```python
from build123d import *

# Parameters (mm, degrees)
BOSS_EXTRUDE1_DEPTH                                  = 4.7625
CUT_EXTRUDE2_DEPTH                                   = 349.730645664
CSK_FOR_M5_CROSS_RECESS_FLAT_HEAD_SCREW1_D           = 3.9624
CSK_FOR_M5_CROSS_RECESS_FLAT_HEAD_SCREW1_CSINK_D     = 6.35
CSK_FOR_M5_CROSS_RECESS_FLAT_HEAD_SCREW1_CSINK_ANGLE = 60
CIRPATTERN1_COUNT                                    = 19
CIRPATTERN1_ANGLE                                    = 45
CBORE_FOR_M5_CROSS_RECESS_PAN_HEAD_SCREW_D           = 4.3434
CBORE_FOR_M5_CROSS_RECESS_PAN_HEAD_SCREW_CBORE_D     = 7.9502
CBORE_FOR_M5_CROSS_RECESS_PAN_HEAD_SCREW_CBORE_DEPTH = 4.1656
CUT_EXTRUDE5_DEPTH                                   = 3.175
F_1_4_20_TAPPED_HOLE1_D                              = 5.1054
F_1_4_20_TAPPED_HOLE1_DEPTH                          = 19.05
F_1_4_20_TAPPED_HOLE1_CSINK_D                        = 7.62
F_1_4_20_TAPPED_HOLE1_CSINK_ANGLE                    = 90
F_1_4_20_TAPPED_HOLE1_TIP                            = 1.533816902


with BuildPart() as part:
    # Sketch1 → Boss-Extrude1 (new, symmetric)
    with BuildSketch(Plane(origin=(0, 0, 0), x_dir=(1, 0, 0), z_dir=(0, 1, 0))):
        with BuildLine():
            Line((38.1, 86.658308315), (238.76, 86.658308315))
            ThreePointArc((238.76, 86.658308315), (135.186201707, 215.036487295), (-25.4, 252.726809025))
            Line((-25.4, 252.726809025), (-25.4, 196.85))
            Line((-25.4, 196.85), (38.1, 133.35))
            Line((38.1, 133.35), (38.1, 86.658308315))
        make_face()
    extrude(amount=BOSS_EXTRUDE1_DEPTH, both=True)

    # Sketch2 → Cut-Extrude2 (cut, through all)
    with BuildSketch(Plane(origin=(0, 4.7625, 0), x_dir=(1, 0, 0), z_dir=(0, 1, 0))):
        with BuildLine():
            ThreePointArc((180.827242585, 147.531326552), (107.760674963, 207.006330595), (17.132342345, 232.74549796))
            ThreePointArc((17.132342345, 232.74549796), (11.965081824, 228.286801882), (16.423777903, 223.119541362))
            ThreePointArc((16.423777903, 223.119541362), (103.303877349, 198.444902033), (173.348536427, 141.429682659))
            ThreePointArc((173.348536427, 141.429682659), (180.138711452, 140.741151526), (180.827242585, 147.531326552))
        make_face()
    extrude(amount=-CUT_EXTRUDE2_DEPTH, mode=Mode.SUBTRACT)

    # CSK for M5 Cross Recess Flat Head Screw1 (through all)
    with Locations(Plane(origin=(0, -4.7625, 0), x_dir=(-1, 0, 0), z_dir=(0, -1, 0))):
        with Locations((-42.342371642, 240.135522494)):
            csk_for_m5_cross_recess_flat_head_screw1 = CounterSinkHole(CSK_FOR_M5_CROSS_RECESS_FLAT_HEAD_SCREW1_D / 2, CSK_FOR_M5_CROSS_RECESS_FLAT_HEAD_SCREW1_CSINK_D / 2, counter_sink_angle=CSK_FOR_M5_CROSS_RECESS_FLAT_HEAD_SCREW1_CSINK_ANGLE)

    # CirPattern1: CSK for M5 Cross Recess Flat Head Screw1 ×19 about axis
    cirpattern1_axis = Axis((0, 0, 0), (0, -1, 0))
    for i in range(1, CIRPATTERN1_COUNT):
        add(csk_for_m5_cross_recess_flat_head_screw1.rotate(cirpattern1_axis, i * CIRPATTERN1_ANGLE / (CIRPATTERN1_COUNT - 1)), mode=Mode.SUBTRACT)

    # CBORE for M5 Cross Recess Pan Head Screw2 (through all)
    with Locations(Plane(origin=(0, -4.7625, 0), x_dir=(-1, 0, 0), z_dir=(0, -1, 0))):
        with Locations((-45.72, 192.1002), (-45.72, 109.5502)):
            CounterBoreHole(CBORE_FOR_M5_CROSS_RECESS_PAN_HEAD_SCREW_D / 2, CBORE_FOR_M5_CROSS_RECESS_PAN_HEAD_SCREW_CBORE_D / 2, CBORE_FOR_M5_CROSS_RECESS_PAN_HEAD_SCREW_CBORE_DEPTH)

    # Sketch10 → Cut-Extrude5 (cut)
    with BuildSketch(Plane(origin=(0, 4.7625, 0), x_dir=(1, 0, 0), z_dir=(0, 1, 0))):
        with BuildLine():
            Line((203.2, 94.532308315), (203.2, 86.658308315))
            Line((203.2, 86.658308315), (212.852, 86.658308315))
            Line((212.852, 86.658308315), (212.852, 94.532308315))
            ThreePointArc((212.852, 94.532308315), (208.026, 99.358308315), (203.2, 94.532308315))
        make_face()
    extrude(amount=-CUT_EXTRUDE5_DEPTH, mode=Mode.SUBTRACT)

    # 1/4-20 Tapped Hole1
    with Locations(Plane.XY.offset(-86.658308315)):
        with Locations((64.77, 0), (144.145, 0), (223.52, 0)):
            CounterSinkHole(F_1_4_20_TAPPED_HOLE1_D / 2, F_1_4_20_TAPPED_HOLE1_CSINK_D / 2, depth=F_1_4_20_TAPPED_HOLE1_DEPTH, counter_sink_angle=F_1_4_20_TAPPED_HOLE1_CSINK_ANGLE)
            with Locations((0, 0, -(F_1_4_20_TAPPED_HOLE1_DEPTH + F_1_4_20_TAPPED_HOLE1_TIP / 2))):  # 118° drill point
                Cone(0, F_1_4_20_TAPPED_HOLE1_D / 2, F_1_4_20_TAPPED_HOLE1_TIP, mode=Mode.SUBTRACT)


solid = part.part
```
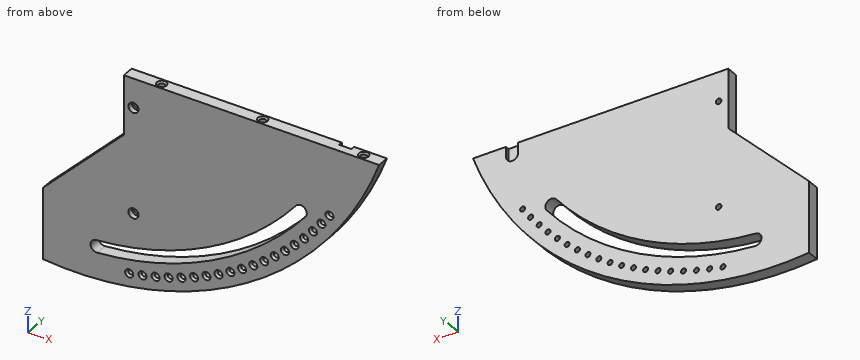
Here's how the part is built. I have some questions about the finished solid (model axes, mm). Coordinates: 2 decimals unless noted, no trailing zeros. Write each loop counter-clockwise with the first axis right and the second up, starting at its lowest first coordinate (ties: lowest second). Pieces come first, ordered by that corner, then holes. Notation, with made-up numbers: M 55,57 L 111,57 A28 ccw 111,82 Z; hole C 44.5,78.25 d5. An arc over 180 degrees is marked long. Answer as CSV lines item,"result". Start each with the question number.
Q1. Will these pins go through, and if not, where does the flat tip stop? pin 1 Ø4.5 at (x, z) = (164.74, -179.78) entering from -Y; pin 2 Ø3 at (x, z) = (206.5, -93) entering from +Y; pin 3 Ø5 at (x, z) = (73.32, -232.55) entering from -Y.
Q2. I need wall thicknesses on probe 1 along Z at (x, y) = (172.5, -0.75); probe 2 along Z at (x, y) = (122, 3); probe 3 along X at (y, z) = (-1.75, -180). Which ranges of each line are inside material? Lowest first, please. Write a range as [from, to].
Q3. Suppose I cut it at A-A, the plane z = -121. List the corners of the cut face in (x, y) for me, then the cut area to 3 significant figures.
Entries:
1,pin 1,"stops at y = -3.17"
1,pin 2,"stops at y = 1.59"
1,pin 3,"stops at y = -3.6"
2,probe 1,"z = [-186.44, -174.4], [-170.44, -157.19], [-142.46, -86.66]"
2,probe 2,"z = [-222.78, -213.15], [-209.19, -198.95], [-187.53, -86.66]"
2,probe 3,"x = [-8.55, 132.86], [148.54, 162.77], [166.7, 179.21]"
3,outline,"M 38.1,-4.76 L 223.33,-4.76 L 223.33,4.76 L 38.1,4.76 Z"
3,area,"1,760 mm²"
